Work out the finished part from the listing and answer in its coordinate system (mm). A direction names the side the tool comes from. Give positions to 0.01 mm unless a question says otherwise; leave off trailing zeros. Loops run counter-clockwise (first coordinate to the right, second up) from the corner with the lowest first, then second, coordinate; pieces in that order, holes last. Notation, with made-up numbers: M -5.5,48 L 24.5,48 A10 cw 24.5,55 Z; hole C 59,76.5 d2. An arc over 180 degrees is marked long. Write item = value, one per line. Start each with the question number.
1. The mould has two halves that part along Y. Classify faces 4 (the face through (-14, -13, 26.4)), 5 (the face through (-14.224, -57.213, -0.035)), 6 (the face through (-14.224, 27.757, 0.469)), 7 (the face through (-14.22, 21.78, 24.59)): released by +Y, released by -Y, zero draft, split by the parting line, or undercut.
2. Section B-B on z = 0 is taken. Determine the outline of the cut face in (x, y).
3. Consider L1, parallel to Z at x = -8, y = -1; L2, parallel to Y at x = -15, z = 2; L3, parallel to Y at x = -18.5, z = -0.5. Determine where each line is inside the solid, lowest interval first. Write a range as [from, to].
4. Flat-ended cylindrical pins translate along their axes: pin 1 Ø9 at (x, z) = (-8.5, -1) entering from +Y; pin 2 Ø1 at (x, z) = (-16, 13) entering from -Y; pin 3 Ø0.6 at (x, z) = (1, -4.5) entering from -Y; pin 4 Ø5 at (x, z) = (-1.5, 7.5) entering from -Y. Find the tip coordinate at first contact, or state that the pin passes through.
5. Section D-D on z = -6 is taken. Determine the outline of the cut face in (x, y), plus the area to 3 significant figures.
6. For faces 1 (the face through (-15.21, -42.64, -19.38)), 2 (the face through (-14.22, 28.4, 11.17)), 3 (the face through (1, 15.187, 0)), determine the directions among +Z, -Z, +X, -X, +Y, -Y from which every point of the face is accessible in a straight line to the end or side of a thin tool.
7. Section A-A on y = -32.5 is taken. Determine the outline of the cut face in (x, z), plus the area to 3 significant figures.
8. Section C-C on x = -12 is taken. Determine the outline of the cut face in (y, z), plus the area to 3 significant figures.
```python
from build123d import *

# Parameters (mm, degrees)
SALIENTE_EXTRUIR1_DEPTH      = 2
SALIENTE_EXTRUIR1_DEPTH_BACK = 30
CROQUIS2_R                   = 3.6
SALIENTE_EXTRUIR2_START      = -2
SALIENTE_EXTRUIR2_DEPTH      = 2


with BuildPart() as part:
    # Croquis2 → Saliente-Extruir1 (new, two sides: drawn at the far end of the back side and taken through both)
    with BuildSketch(Plane(origin=(0, 0, 0), x_dir=(0, 0, -1), z_dir=(1, 0, 0)).offset(-SALIENTE_EXTRUIR1_DEPTH_BACK)):
        with BuildLine():
            Line((-26.4, -41.464925013), (-26.4, 16.039678623))
            ThreePointArc((-26.4, 16.039678623), (-24.535471531, 21.85466813), (-19.637179406, 25.501214941))
            Line((-19.637179406, 25.501214941), (-2.460256349, 31.378144407))
            ThreePointArc((-2.460256349, 31.378144407), (0, 31.787376805), (2.460256349, 31.378144407))
            Line((2.460256349, 31.378144407), (19.637179406, 25.501214941))
            ThreePointArc((19.637179406, 25.501214941), (24.535471531, 21.85466813), (26.4, 16.039678623))
            Line((26.4, 16.039678623), (26.4, -41.464925013))
            ThreePointArc((26.4, -41.464925013), (24.535471531, -47.27991452), (19.637179406, -50.92646133))
            Line((19.637179406, -50.92646133), (2.460256349, -56.803390796))
            ThreePointArc((2.460256349, -56.803390796), (0, -57.212623195), (-2.460256349, -56.803390796))
            Line((-2.460256349, -56.803390796), (-19.637179406, -50.92646133))
            ThreePointArc((-19.637179406, -50.92646133), (-24.535471531, -47.27991452), (-26.4, -41.464925013))
        make_face()
        with Locations((0, 24.187376805)):
            Circle(CROQUIS2_R, mode=Mode.SUBTRACT)
        with Locations(Location((0, -49.612623195, 0), (0, 0, 180))):
            Circle(CROQUIS2_R, mode=Mode.SUBTRACT)
        with BuildLine():
            Line((20.4, -40.212623195), (20.4, 14.787376805))
            ThreePointArc((20.4, 14.787376805), (19.404163056, 17.191539861), (17, 18.187376805))
            Line((17, 18.187376805), (0, 18.187376805))
            Line((0, 18.187376805), (-17, 18.187376805))
            ThreePointArc((-17, 18.187376805), (-19.404163056, 17.191539861), (-20.4, 14.787376805))
            Line((-20.4, 14.787376805), (-20.4, -40.212623195))
            ThreePointArc((-20.4, -40.212623195), (-19.404163056, -42.616786251), (-17, -43.612623195))
            Line((-17, -43.612623195), (0, -43.612623195))
            Line((0, -43.612623195), (17, -43.612623195))
            ThreePointArc((17, -43.612623195), (19.404163056, -42.616786251), (20.4, -40.212623195))
        make_face(mode=Mode.SUBTRACT)
    extrude(amount=SALIENTE_EXTRUIR1_DEPTH + SALIENTE_EXTRUIR1_DEPTH_BACK)

    # Croquis3 → Saliente-Extruir2 (add)
    with BuildSketch(Plane(origin=(2, 0, 0), x_dir=(0, 0, -1), z_dir=(1, 0, 0)).offset(SALIENTE_EXTRUIR2_START)):
        with BuildLine():
            Line((-17, -43.612623195), (17, -43.612623195))
            ThreePointArc((17, -43.612623195), (19.404163056, -42.616786251), (20.4, -40.212623195))
            Line((20.4, -40.212623195), (20.4, 14.787376805))
            ThreePointArc((20.4, 14.787376805), (19.404163056, 17.191539861), (17, 18.187376805))
            Line((17, 18.187376805), (-17, 18.187376805))
            ThreePointArc((-17, 18.187376805), (-19.404163056, 17.191539861), (-20.4, 14.787376805))
            Line((-20.4, 14.787376805), (-20.4, -40.212623195))
            ThreePointArc((-20.4, -40.212623195), (-19.404163056, -42.616786251), (-17, -43.612623195))
        make_face()
        with BuildLine():
            Line((-17, -40.612623195), (17, -40.612623195))
            ThreePointArc((17, -40.612623195), (17.282842712, -40.495465907), (17.4, -40.212623195))
            Line((17.4, -40.212623195), (17.4, 14.787376805))
            ThreePointArc((17.4, 14.787376805), (17.282842712, 15.070219518), (17, 15.187376805))
            Line((17, 15.187376805), (-17, 15.187376805))
            ThreePointArc((-17, 15.187376805), (-17.282842712, 15.070219518), (-17.4, 14.787376805))
            Line((-17.4, 14.787376805), (-17.4, -40.212623195))
            ThreePointArc((-17.4, -40.212623195), (-17.282842712, -40.495465907), (-17, -40.612623195))
        make_face(mode=Mode.SUBTRACT)
    extrude(amount=SALIENTE_EXTRUIR2_DEPTH)


solid = part.part
```
Verdict:
q1.face_4 = zero draft
q1.face_5 = released by -Y
q1.face_6 = undercut
q1.face_7 = released by +Y
q2.outline = M -30,-57.21 L 2,-57.21 L 2,-53.21 L -30,-53.21 Z; M -30,-46.01 L 2,-46.01 L 2,-40.61 L 0,-40.61 L 0,-43.61 L -30,-43.61 Z; M -30,18.19 L 0,18.19 L 0,15.19 L 2,15.19 L 2,20.59 L -30,20.59 Z; M -30,27.79 L 2,27.79 L 2,31.79 L -30,31.79 Z
q3.L1 = [-26.4, -20.4], [20.4, 26.4]
q3.L2 = [-56.94, -52.61], [-46.62, -43.61], [18.19, 21.19], [27.18, 31.52]
q3.L3 = [-57.2, -53.18], [-46.05, -43.61], [18.19, 20.62], [27.75, 31.77]
q4.pin_1 = 31.79
q4.pin_2 = -53.37
q4.pin_3 = -56.21
q4.pin_4 = -55.93
q5.outline = M -30,-55.59 L 2,-55.59 L 2,-40.61 L 0,-40.61 L 0,-43.61 L -30,-43.61 Z; M -30,18.19 L 0,18.19 L 0,15.19 L 2,15.19 L 2,30.17 L -30,30.17 Z
q5.area = 779 mm2
q6.face_1 = -X
q6.face_2 = +Z, +X, -X, +Y
q6.face_3 = +X, -X
q7.outline = M -30,-26.4 L 2,-26.4 L 2,-17.4 L 0,-17.4 L 0,-20.4 L -30,-20.4 Z; M -30,20.4 L 0,20.4 L 0,17.4 L 2,17.4 L 2,26.4 L -30,26.4 Z
q7.area = 396 mm2
q8.outline = M -56.8,-2.46 L -50.93,-19.64 A10 ccw -41.46,-26.4 L 16.04,-26.4 A10 ccw 25.5,-19.64 L 31.38,-2.46 A7.6 ccw 31.38,2.46 L 25.5,19.64 A10 ccw 16.04,26.4 L -41.46,26.4 A10 ccw -50.93,19.64 L -56.8,2.46 A7.6 ccw Z; hole C -49.61,0 d7.2; hole M -43.61,-17 A3.4 ccw -40.21,-20.4 L 14.79,-20.4 A3.4 ccw 18.19,-17 L 18.19,17 A3.4 ccw 14.79,20.4 L -40.21,20.4 A3.4 ccw -43.61,17 Z; hole C 24.19,0 d7.2
q8.area = 1,640 mm2
